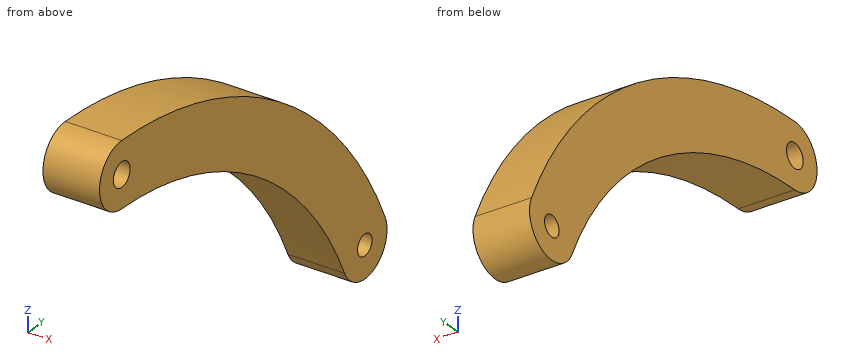
from build123d import *

# Parameters (mm, degrees)
ESQUISSE1_R        = 1.190625
ESQUISSE1_R_2      = 1.031875
BOSS_EXTRU_1_DEPTH = 5.588


with BuildPart() as part:
    # Esquisse1 → Boss.-Extru.1 (new body)
    with BuildSketch(Plane(origin=(0, 0, 0), x_dir=(0, 0, -1), z_dir=(1, 0, 0))):
        with BuildLine():
            ThreePointArc((-34.925, 0), (-29.357723625, 18.917708333), (-14.430815972, 31.804200593))
            ThreePointArc((-14.430815972, 31.804200593), (-12.85141737, 36.007383917), (-17.054600694, 37.586782519))
            ThreePointArc((-17.054600694, 37.586782519), (-34.695491556, 22.357291667), (-41.275, 0))
            ThreePointArc((-41.275, 0), (-38.1, -3.175), (-34.925, 0))
        make_face()
        with Locations((-38.1, 0)):
            Circle(ESQUISSE1_R, mode=Mode.SUBTRACT)
        with Locations((-15.742708333, 34.695491556)):
            Circle(ESQUISSE1_R_2, mode=Mode.SUBTRACT)
    extrude(amount=BOSS_EXTRU_1_DEPTH)


solid = part.part
Model file for the job. Use its own axes, mm. Give positions to 0.01 mm unless a question says otherwise; leave off trailing zeros. Order: outer loops, then holes, each group sorted by start corner. A loop starts at its lowest first (then second) coordinate and runs counter-clockwise, first axis right, second up. Notation, with made-up numbers: (1.5, 39.5) - (44.5, 39.5) arc R28 cw to (44.5, 73.5) - close; hole circle Ø7 at (-21, 43). An arc over 180 degrees is marked (long way). One line per item, written item: value.
Item 1: Slice it at D-D (z = 16). List the corners of the cut face in (x, y).
Response values:
outline: (0, 31.04) - (5.59, 31.04) - (5.59, 33.7) - (0, 33.7) - close; (0, 35.69) - (5.59, 35.69) - (5.59, 37.86) - (0, 37.86) - close
Item 2: Slice it at B-B (x = 4.6). Give the number of separate pieces and of enclosed holes in the cut face, then the cut area to 3 significant figures.
Response values:
separate pieces: 1
enclosed holes: 2
area: 301 mm2
Item 3: Wall check: line 1 (Y direction, x = 5.35, z = 15.75); line 2 (Y direction, x = 3.9, z = 38.1) (3 decimals); line 3 (Z direction, x = 1.8, y = 11.5). Give the ranges that are in metal, low to high.
Response values:
line 1: 31.17 to 33.66, 35.73 to 37.87
line 2: -3.175 to -1.191, 1.191 to 15.875
line 3: 32.98 to 39.64
Item 4: Slice it at A-A (z = 38.1). List the corners of the cut face in (x, y) (3 decimals).
Response values:
outline: (0, -3.175) - (5.588, -3.175) - (5.588, -1.191) - (0, -1.191) - close; (0, 1.191) - (5.588, 1.191) - (5.588, 15.875) - (0, 15.875) - close
Item 5: Slice it at C-C (y = 6.5). List the corners of the cut face in (x, z), then the cut area to 3 significant figures.
Response values:
outline: (0, 34.31) - (5.59, 34.31) - (5.59, 40.76) - (0, 40.76) - close
area: 36.0 mm2
Item 6: Pin check, flat tip, straight feed: pin 1 Ø3 at (x, z) = (1, 33.5) entering from +Y. Stop position of the tip, or through.
Response values:
pin 1: y = 26.07
